Autodesk Inventor part; units mm, degrees
ref_plane "YZ Plane" through (0, 0, 0) normal (1, 0, 0) x (0, 1, 0)
ref_plane "XZ Plane" through (0, 0, 0) normal (0, 1, 0) x (-1, 0, 0)
ref_plane "XY Plane" through (0, 0, 0) normal (0, 0, 1) x (1, 0, 0)
sketch "Sketch1" plane through (0, 0, 0) normal (0, 0, 1) x (1, 0, 0)
  line L0 (-10, -10) -> (10, 10) construction
  line L1 (10, -10) -> (-10, 10) construction
  arc A0 (-10, -9.5) -> (-9.5, -10) centre (-9.5, -9.5) ccw
  arc A1 (-9.5, 10) -> (-10, 9.5) centre (-9.5, 9.5) ccw
  arc A2 (10, 9.5) -> (9.5, 10) centre (9.5, 9.5) ccw
  arc A3 (9.5, -10) -> (10, -9.5) centre (9.5, -9.5) ccw
  line L2 (7, -7) -> (-7, -7) construction
  line L3 (-7, -7) -> (-7, 7) construction
  line L4 (-7, 7) -> (7, 7) construction
  line L5 (7, 7) -> (7, -7) construction
  line L6 (7, -7) -> (-7, 7) construction
  line L7 (-7, -7) -> (7, 7) construction
  circle A4 centre (-7, -7) radius 2
  circle A5 centre (-7, 7) radius 2
  circle A6 centre (7, 7) radius 2
  circle A7 centre (7, -7) radius 2
  circle A8 centre (0, 0) radius 2.15
  line L8 (-8.5, 4.15) -> (-5.1906, 4.15)
  arc A9 (-5.1906, -4.15) -> (-5.1906, 4.15) centre (-8.8, 0) ccw
  line L9 (-5.1906, -4.15) -> (-8.5, -4.15)
  line L10 (-8.5, -4.15) -> (-8.5, -2.7559)
  line L11 (-8.5, 2.5441) -> (-8.5, 4.15)
  line L12 (-5.1906, -4.15) -> (-5.1906, 4.15) construction
  line L13 (-8.5, -2.7559) -> (-10, -2.7559)
  line L14 (-8.5, 2.5441) -> (-10, 2.5441)
  line L15 (-10, 9.5) -> (-10, 2.5441)
  line L16 (-10, -2.7559) -> (-10, -9.5)
  line L17 (4.15, -8.5) -> (2.7559, -8.5)
  line L18 (2.7559, -8.5) -> (2.7559, -10)
  line L19 (4.15, -5.1906) -> (-4.15, -5.1906) construction
  arc A10 (4.15, -5.1906) -> (-4.15, -5.1906) centre (0, -8.8) ccw
  line L20 (7, -7) -> (-7, 7) construction
  line L21 (10, -10) -> (-10, 10) construction
  line L22 (-4.15, -8.5) -> (-4.15, -5.1906)
  line L23 (4.15, -5.1906) -> (4.15, -8.5)
  line L24 (-2.5441, -8.5) -> (-2.5441, -10)
  line L25 (-2.5441, -8.5) -> (-4.15, -8.5)
  line L26 (8.5, 4.15) -> (8.5, 2.7559)
  line L27 (8.5, 2.7559) -> (10, 2.7559)
  line L28 (5.1906, 4.15) -> (5.1906, -4.15) construction
  arc A11 (5.1906, 4.15) -> (5.1906, -4.15) centre (8.8, 0) ccw
  line L29 (7, 7) -> (-7, -7) construction
  line L30 (10, 10) -> (-10, -10) construction
  line L31 (8.5, -4.15) -> (5.1906, -4.15)
  line L32 (5.1906, 4.15) -> (8.5, 4.15)
  line L33 (8.5, -2.5441) -> (10, -2.5441)
  line L34 (8.5, -2.5441) -> (8.5, -4.15)
  line L35 (-4.15, 8.5) -> (-2.7559, 8.5)
  line L36 (-2.7559, 8.5) -> (-2.7559, 10)
  line L37 (-4.15, 5.1906) -> (4.15, 5.1906) construction
  arc A12 (-4.15, 5.1906) -> (4.15, 5.1906) centre (0, 8.8) ccw
  line L38 (-7, 7) -> (7, -7) construction
  line L39 (-10, 10) -> (10, -10) construction
  line L40 (4.15, 8.5) -> (4.15, 5.1906)
  line L41 (-4.15, 5.1906) -> (-4.15, 8.5)
  line L42 (2.5441, 8.5) -> (2.5441, 10)
  line L43 (2.5441, 8.5) -> (4.15, 8.5)
  line L44 (-9.5, -10) -> (-2.5441, -10)
  line L45 (2.7559, -10) -> (9.5, -10)
  line L46 (9.5, 10) -> (2.5441, 10)
  line L47 (-2.7559, 10) -> (-9.5, 10)
  line L48 (10, -9.5) -> (10, -2.5441)
  line L49 (10, 2.7559) -> (10, 9.5)
  line L50 (2292.4151, 1187.1915) -> (2314.8128, 1187.1915)
  circle A13 centre (2303.6139, 1187.1915) radius 2.15
  line L51 (2307.7639, 1192.1343) -> (2307.7639, 1195.3915)
  arc A14 (2307.7639, 1195.3915) -> (2307.4639, 1195.6915) centre (2307.4639, 1195.3915) ccw
  line L52 (2307.4639, 1195.6915) -> (2306.5639, 1195.6915)
  arc A15 (2306.2639, 1195.9915) -> (2306.5639, 1195.6915) centre (2306.5639, 1195.9915) ccw
  line L53 (2306.2639, 1195.9915) -> (2306.2639, 1196.8915)
  arc A16 (2306.5639, 1197.1915) -> (2306.2639, 1196.8915) centre (2306.5639, 1196.8915) ccw
  line L54 (2306.5639, 1197.1915) -> (2313.3139, 1197.1915)
  arc A17 (2313.6139, 1196.8915) -> (2313.3139, 1197.1915) centre (2313.3139, 1196.8915) ccw
  line L55 (2313.6139, 1196.8915) -> (2313.6139, 1190.1415)
  arc A18 (2313.3139, 1189.8415) -> (2313.6139, 1190.1415) centre (2313.3139, 1190.1415) ccw
  line L56 (2313.3139, 1189.8415) -> (2312.4139, 1189.8415)
  arc A19 (2312.1139, 1190.1415) -> (2312.4139, 1189.8415) centre (2312.4139, 1190.1415) ccw
  line L57 (2312.1139, 1190.1415) -> (2312.1139, 1191.0415)
  arc A20 (2312.1139, 1191.0415) -> (2311.8139, 1191.3415) centre (2311.8139, 1191.0415) ccw
  line L58 (2311.8139, 1191.3415) -> (2308.5567, 1191.3415)
  arc A21 (2308.5567, 1191.3415) -> (2308.3217, 1191.2281) centre (2308.5567, 1191.0415) ccw
  arc A22 (2308.3217, 1191.2281) -> (2306.9212, 1187.4988) centre (2313.4048, 1187.1915) ccw
  line L59 (2306.9212, 1187.4988) -> (2306.6139, 1187.1915)
  line L60 (2306.6139, 1187.1915) -> (2306.9212, 1186.8843)
  arc A23 (2306.9212, 1186.8843) -> (2308.3217, 1183.155) centre (2313.4048, 1187.1915) ccw
  arc A24 (2308.3217, 1183.155) -> (2308.5567, 1183.0415) centre (2308.5567, 1183.3415) ccw
  line L61 (2308.5567, 1183.0415) -> (2311.8139, 1183.0415)
  arc A25 (2311.8139, 1183.0415) -> (2312.1139, 1183.3415) centre (2311.8139, 1183.3415) ccw
  line L62 (2312.1139, 1183.3415) -> (2312.1139, 1184.2415)
  arc A26 (2312.4139, 1184.5415) -> (2312.1139, 1184.2415) centre (2312.4139, 1184.2415) ccw
  line L63 (2312.4139, 1184.5415) -> (2313.3139, 1184.5415)
  arc A27 (2313.6139, 1184.2415) -> (2313.3139, 1184.5415) centre (2313.3139, 1184.2415) ccw
  line L64 (2313.6139, 1184.2415) -> (2313.6139, 1177.4915)
  arc A28 (2313.3139, 1177.1915) -> (2313.6139, 1177.4915) centre (2313.3139, 1177.4915) ccw
  line L65 (2313.3139, 1177.1915) -> (2306.5639, 1177.1915)
  arc A29 (2306.2639, 1177.4915) -> (2306.5639, 1177.1915) centre (2306.5639, 1177.4915) ccw
  line L66 (2306.2639, 1177.4915) -> (2306.2639, 1178.3915)
  arc A30 (2306.5639, 1178.6915) -> (2306.2639, 1178.3915) centre (2306.5639, 1178.3915) ccw
  line L67 (2306.5639, 1178.6915) -> (2307.4639, 1178.6915)
  arc A31 (2307.4639, 1178.6915) -> (2307.7639, 1178.9915) centre (2307.4639, 1178.9915) ccw
  line L68 (2307.7639, 1178.9915) -> (2307.7639, 1182.2488)
  arc A32 (2307.7639, 1182.2488) -> (2307.6505, 1182.4837) centre (2307.4639, 1182.2488) ccw
  arc A33 (2307.6505, 1182.4837) -> (2303.9212, 1183.8843) centre (2303.6139, 1177.4007) ccw
  line L69 (2303.9212, 1183.8843) -> (2303.6139, 1184.1915)
  line L70 (2303.6139, 1184.1915) -> (2303.3066, 1183.8843)
  arc A34 (2303.3066, 1183.8843) -> (2299.5774, 1182.4837) centre (2303.6139, 1177.4007) ccw
  arc A35 (2299.5774, 1182.4837) -> (2299.4639, 1182.2488) centre (2299.7639, 1182.2488) ccw
  line L71 (2299.4639, 1182.2488) -> (2299.4639, 1178.9915)
  arc A36 (2299.4639, 1178.9915) -> (2299.7639, 1178.6915) centre (2299.7639, 1178.9915) ccw
  line L72 (2299.7639, 1178.6915) -> (2300.6639, 1178.6915)
  arc A37 (2300.9639, 1178.3915) -> (2300.6639, 1178.6915) centre (2300.6639, 1178.3915) ccw
  line L73 (2300.9639, 1178.3915) -> (2300.9639, 1177.4915)
  arc A38 (2300.6639, 1177.1915) -> (2300.9639, 1177.4915) centre (2300.6639, 1177.4915) ccw
  line L74 (2300.6639, 1177.1915) -> (2293.9139, 1177.1915)
  arc A39 (2293.6139, 1177.4915) -> (2293.9139, 1177.1915) centre (2293.9139, 1177.4915) ccw
  line L75 (2293.6139, 1177.4915) -> (2293.6139, 1184.2415)
  arc A40 (2293.9139, 1184.5415) -> (2293.6139, 1184.2415) centre (2293.9139, 1184.2415) ccw
  line L76 (2293.9139, 1184.5415) -> (2294.8139, 1184.5415)
  arc A41 (2295.1139, 1184.2415) -> (2294.8139, 1184.5415) centre (2294.8139, 1184.2415) ccw
  line L77 (2295.1139, 1184.2415) -> (2295.1139, 1183.3415)
  arc A42 (2295.1139, 1183.3415) -> (2295.4139, 1183.0415) centre (2295.4139, 1183.3415) ccw
  line L78 (2295.4139, 1183.0415) -> (2298.6712, 1183.0415)
  arc A43 (2298.6712, 1183.0415) -> (2298.9061, 1183.155) centre (2298.6712, 1183.3415) ccw
  arc A44 (2298.9061, 1183.155) -> (2300.3066, 1186.8843) centre (2293.8231, 1187.1915) ccw
  line L79 (2300.3066, 1186.8843) -> (2300.6139, 1187.1915)
  line L80 (2300.6139, 1187.1915) -> (2300.3066, 1187.4988)
  arc A45 (2300.3066, 1187.4988) -> (2298.9061, 1191.2281) centre (2293.8231, 1187.1915) ccw
  arc A46 (2298.9061, 1191.2281) -> (2298.6712, 1191.3415) centre (2298.6712, 1191.0415) ccw
  line L81 (2298.6712, 1191.3415) -> (2295.4139, 1191.3415)
  arc A47 (2295.4139, 1191.3415) -> (2295.1139, 1191.0415) centre (2295.4139, 1191.0415) ccw
  line L82 (2295.1139, 1191.0415) -> (2295.1139, 1190.1415)
  arc A48 (2294.8139, 1189.8415) -> (2295.1139, 1190.1415) centre (2294.8139, 1190.1415) ccw
  line L83 (2294.8139, 1189.8415) -> (2293.9139, 1189.8415)
  arc A49 (2293.6139, 1190.1415) -> (2293.9139, 1189.8415) centre (2293.9139, 1190.1415) ccw
  line L84 (2293.6139, 1190.1415) -> (2293.6139, 1196.8915)
  arc A50 (2293.9139, 1197.1915) -> (2293.6139, 1196.8915) centre (2293.9139, 1196.8915) ccw
  line L85 (2293.9139, 1197.1915) -> (2300.6639, 1197.1915)
  arc A51 (2300.9639, 1196.8915) -> (2300.6639, 1197.1915) centre (2300.6639, 1196.8915) ccw
  line L86 (2300.9639, 1196.8915) -> (2300.9639, 1195.9915)
  arc A52 (2300.6639, 1195.6915) -> (2300.9639, 1195.9915) centre (2300.6639, 1195.9915) ccw
  line L87 (2300.6639, 1195.6915) -> (2299.7639, 1195.6915)
  arc A53 (2299.7639, 1195.6915) -> (2299.4639, 1195.3915) centre (2299.7639, 1195.3915) ccw
  line L88 (2299.4639, 1195.3915) -> (2299.4639, 1192.1343)
  arc A54 (2299.4639, 1192.1343) -> (2299.5774, 1191.8994) centre (2299.7639, 1192.1343) ccw
  arc A55 (2299.5774, 1191.8994) -> (2303.3066, 1190.4988) centre (2303.6139, 1196.9824) ccw
  line L89 (2303.3066, 1190.4988) -> (2303.6139, 1190.1915)
  line L90 (2303.6139, 1190.1915) -> (2303.9212, 1190.4988)
  arc A56 (2303.9212, 1190.4988) -> (2307.6505, 1191.8994) centre (2303.6139, 1196.9824) ccw
  arc A57 (2307.6505, 1191.8994) -> (2307.7639, 1192.1343) centre (2307.4639, 1192.1343) ccw
  line L91 (2294.1139, 1194.1915) -> (2299.1139, 1194.1915)
  line L92 (2296.6139, 1196.6915) -> (2296.6139, 1191.6915)
  circle A58 centre (2296.6139, 1194.1915) radius 2
  line L93 (2294.1139, 1180.1915) -> (2299.1139, 1180.1915)
  line L94 (2296.6139, 1177.6915) -> (2296.6139, 1182.6915)
  circle A59 centre (2296.6139, 1180.1915) radius 2
  line L95 (2303.6139, 1198.3904) -> (2303.6139, 1175.9927)
  line L96 (2313.1139, 1194.1915) -> (2308.1139, 1194.1915)
  line L97 (2310.6139, 1196.6915) -> (2310.6139, 1191.6915)
  circle A60 centre (2310.6139, 1194.1915) radius 2
  circle A61 centre (2310.6139, 1180.1915) radius 2
  line L98 (2310.6139, 1177.6915) -> (2310.6139, 1182.6915)
  line L99 (2313.1139, 1180.1915) -> (2308.1139, 1180.1915)
  point P0 (-10, 0)
  point P1 (-5.8595, 0)
  point P2 (-5.1906, 0)
  point P3 (-10, 0)
  point P4 (0, -5.8595)
  point P5 (0, -5.1906)
  point P6 (5.8595, 0)
  point P7 (5.1906, 0)
  point P8 (0, 5.8595)
  point P9 (0, 5.1906)
  dimension "d0" = 20
  dimension "d1" = 20
  dimension "d2" = 0.5
  dimension "d3" = 14
  dimension "d4" = 14
  dimension "d5" = 4
  dimension "d6" = 4.3
  dimension "d13" = 5.5
  dimension "d14" = 8.3
  dimension "d16" = 5.3
  dimension "d17" = 6.7
  dimension "d18" = 1.5
  dimension "d21" = 360
extrude "Extrusion1" add sketch "Sketch1" along normal blind 276 contours L16 L13 L10 L9 A9 L8 L11 L14 L15 A1 L47 L36 L35 L41 A12 L40 L43 L42 L46 A2 L49 L27 L26 L32 A11 L31 L34 L33 L48 A3 L45 L18 L17 L23 A10 L22 L25 L24 L44 A0
properties part number "Profile_CPY2"
For this review, take the finished solid that the model builds, in its own axes (mm). A direction names the side the tool comes from. Coordinates: 2 decimals unless noted, no trailing zeros.
1. Mouldability with a two-part tool opening along Y and no side actions: class faces 3 (the flat face through (-2.4, 0.1, 276)), 4 (the cylindrical face through (0.1, 3.3, 136.1)), 5 (the flat face through (-6, 10, 136)) as +Y half, -Y half, draft (parallel to the pull), parting line (faces both ways), or undercut.
2. For faces 1 (the flat face through (6, 10, 136)), 2 (the cylindrical face through (-0.1, -3.3, 136.1)), list the 3-axis set-ups (+Z, -Z, +X, -X, +Y, -Y) from which the entire face can be reached by the end or side of a thin tool; tool diameter is ignored.
3. Insertion check: P1, Ø5, axis at y = 0, z = 125, coming from the +X side. The pin has a flat end and moves straight along its axis. Give the tip position at first contact, or say it passes through.
4. For line 1 (Y direction, x = 7, z = 188); line 2 (X direction, y = 6, z = 34.5); line 3 (Y direction, x = 6.5, z = 90.5), list the stretches that pass through material, from the lowest coordinate up.
5. Add section A-A, the plane z = 20.5. Count the separate pieces of the cut face and the enclosed holes in it, then the cut area to 3 significant figures.
Result:
1. face 3: draft
1. face 4: undercut
1. face 5: +Y half
2. face 1: +Z, -Z, +X, -X, +Y
2. face 2: +Z, -Z
3. P1: stops at x = 3.9
4. line 1: y = -10 to -9, -5 to -4.15, 4.15 to 5, 9 to 10
4. line 2: x = -10 to -8.73, -5.27 to -4.15, 4.15 to 5.27, 8.73 to 10
4. line 3: y = -10 to -8.94, -5.06 to -4.15, 4.15 to 5.06, 8.94 to 10
5. separate pieces: 1
5. enclosed holes: 5
5. area: 150 mm2
